Geometry: final body of the model. Coordinates: model frame, mm. A direction names the side the tool comes from. Round coordinates to 2 decimals unless told otherwise and drop trailing zeros. Loops run counter-clockwise (first coordinate to the right, second up) from the corner with the lowest first, then second, coordinate; pieces in that order, holes last. Notation, with made-up numbers: M -33.75,-1 L -17.75,-1 A26 cw -17.75,17 Z; hole C -14.75,6.5 d5. An arc over 180 degrees is marked long. Answer as a JSON object with one key per item and string values.
from build123d import *

# Parameters (mm, degrees)
BOARDSKE_R   = 0.5
BOARDSKE_R_2 = 3.75
BOARD_DEPTH  = 1
FILLET_2_R   = 1


with BuildPart() as part:
    # BoardSke → Board (new body)
    with BuildSketch(Plane.XY):
        Polygon((9, 13), (9, 9.5), (20.5, 9.5), (20.5, -9.5), (-9, -9.5), (-9, 13), align=None)
        with Locations((-6, 0)):
            Circle(BOARDSKE_R, mode=Mode.SUBTRACT)
        Circle(BOARDSKE_R_2, mode=Mode.SUBTRACT)
        with Locations((3, 5.196152423)):
            Circle(BOARDSKE_R, mode=Mode.SUBTRACT)
        with Locations((3, -5.196152423)):
            Circle(BOARDSKE_R, mode=Mode.SUBTRACT)
    extrude(amount=BOARD_DEPTH)

    # Fillet 2
    fillet_2_edges = [part.edges().sort_by_distance(p)[0] for p in [
        (9, 13, 0.5),
        (9, 9.5, 0.5),
        (20.5, 9.5, 0.5),
        (20.5, -9.5, 0.5),
        (-9, -9.5, 0.5),
        (-9, 13, 0.5),
    ]]
    fillet(fillet_2_edges, radius=FILLET_2_R)


solid = part.part
1) Pin query (flat end, axial travel): P1, Ø6, axis at x = 0, y = 0, coming from the +Z side. Return the tip coordinate at first contact, or that it passes through.
Results:
{"P1": "through"}
2) Pull-direction query (Y, two-part tool) for faces 1 (the flat face through (5.9, -9.5, 0.5)), 2 (the cylindrical face through (9.285, 9.801, 0.507)), 3 (the cylindrical face through (-3.746, 0.165, 0.493)), 4 (the flat face through (6, 2, 0)); classes: +Y half, -Y half, draft (parallel to the pull), parting line (faces both ways), or undercut.
Results:
{"face 1": "-Y half", "face 2": "+Y half", "face 3": "undercut", "face 4": "draft"}
3) Section query B-B (x = -6). Return the cut outline in (y, z), and give its area (3 significant figures).
Results:
{"outline": "M -9.5,0 L -0.5,0 L -0.5,1 L -9.5,1 Z; M 0.5,0 L 13,0 L 13,1 L 0.5,1 Z", "area": "21.5 mm2"}
4) Section query D-D (x = 3). Return the cut outline in (y, z).
Results:
{"outline": "M -9.5,0 L -5.7,0 L -5.7,1 L -9.5,1 Z; M -4.7,0 L -2.25,0 L -2.25,1 L -4.7,1 Z; M 2.25,0 L 4.7,0 L 4.7,1 L 2.25,1 Z; M 5.7,0 L 13,0 L 13,1 L 5.7,1 Z"}
5) Ray query, line 1 (Y direction, x = -6, z = 0.3); line 2 (Y direction, x = 0, z = 0.7); line 3 (X direction, y = 2.5, z = 0.3). Return the intervals inside material, ascending.
Results:
{"line 1": "-9.5 to -0.5, 0.5 to 13", "line 2": "-9.5 to -3.75, 3.75 to 13", "line 3": "-9 to -2.8, 2.8 to 20.5"}
6) Section query A-A (y = -2.25). Return the cut outline in (x, z).
Results:
{"outline": "M -9,0 L -3,0 L -3,1 L -9,1 Z; M 3,0 L 20.5,0 L 20.5,1 L 3,1 Z"}
7) Reachability of faces 5 (the flat face through (14.7, 9.5, 0.5)), 6 (the cylindrical face through (2.5, 5.2, 0.5)) from +Z, -Z, +X, -X, +Y, -Y: full face, straight path, thin tool, end or side. Return the list, or none.
Results:
{"face 5": "+Z, -Z, +X, +Y", "face 6": "+Z, -Z"}
8) Section query C-C (y = 0). Return the cut outline in (x, z).
Results:
{"outline": "M -9,0 L -6.5,0 L -6.5,1 L -9,1 Z; M -5.5,0 L -3.75,0 L -3.75,1 L -5.5,1 Z; M 3.75,0 L 20.5,0 L 20.5,1 L 3.75,1 Z"}
